from build123d import *

# Parameters (mm, degrees)
SKETCH012_W     = 64
SKETCH012_H     = 31
PAD006_DEPTH    = 3
SKETCH013_R     = 1.5
POCKET006_DEPTH = 5
SKETCH014_W     = 8
SKETCH014_H     = 6
POCKET007_DEPTH = 5


with BuildPart() as part:
    # Sketch012 → Pad006 (new body)
    with BuildSketch(Plane.XZ.offset(-30)):
        with Locations((0, -2)):
            Rectangle(SKETCH012_W, SKETCH012_H)
    extrude(amount=PAD006_DEPTH)

    # Sketch013 (on Face5 of Pad006) → Pocket006 (cut)
    with BuildSketch(Plane(origin=(0, 30, 0), x_dir=(1, 0, 0), z_dir=(0, 1, 0))):
        with Locations((28.5, 10)):
            Circle(SKETCH013_R)
        with Locations((-28.5, 10)):
            Circle(SKETCH013_R)
    extrude(amount=-POCKET006_DEPTH, mode=Mode.SUBTRACT)

    # Sketch014 (on Face5 of Pocket006) → Pocket007 (cut)
    with BuildSketch(Plane.XZ.offset(-27)):
        with Locations((19.4, -6)):
            Rectangle(SKETCH014_W, SKETCH014_H)
        with Locations((-0.5, -12)):
            Rectangle(SKETCH014_W, SKETCH014_H)
        with Locations((-19.4, -6)):
            Rectangle(SKETCH014_W, SKETCH014_H)
    extrude(amount=-POCKET007_DEPTH, mode=Mode.SUBTRACT)


with BuildPart() as part_1:
    # Body004 placement: moved
    add(part.part.moved(Location((0, -57, 0))))


solid = part_1.part
For this review, take the finished solid that the model builds, in its own axes (mm). A direction names the side the tool comes from. Round coordinates to 2 decimals unless told otherwise and drop trailing zeros. Loops run counter-clockwise (first coordinate to the right, second up) from the corner with the lowest first, then second, coordinate; pieces in that order, holes last. Notation, with made-up numbers: (-18, 55.25) - (27, 55.25) arc R21 cw to (27, 91.25) - close; hole circle Ø11 at (22.5, 53.25). An arc over 180 degrees is marked (long way). Use one line per item in the form item = value.
Item 1: Consider section D-D on y = -29.1. Write out the cut boundary in (x, z), then the cut area to 3 significant figures.
Answers:
outline = (-32, -17.5) - (32, -17.5) - (32, 13.5) - (-32, 13.5) - close; hole circle Ø3 at (-28.5, -10); hole (-23.4, -9) - (-15.4, -9) - (-15.4, -3) - (-23.4, -3) - close; hole (-4.5, -15) - (3.5, -15) - (3.5, -9) - (-4.5, -9) - close; hole (15.4, -9) - (23.4, -9) - (23.4, -3) - (15.4, -3) - close; hole circle Ø3 at (28.5, -10)
area = 1,830 mm^2
Item 2: Consider section A-A on x = -19.5. Write out the cut boundary in (y, z).
Answers:
outline = (-30, -17.5) - (-27, -17.5) - (-27, -9) - (-30, -9) - close; (-30, -3) - (-27, -3) - (-27, 13.5) - (-30, 13.5) - close
Item 3: Clearance check with a flat-ended pin moving along its axis: P1, Ø1.8, axis at x = -28.5, z = -10, coming from the +Y side. State where the tip first meets the part, or that it passes through.
Answers:
P1 = through
Item 4: For line 1 (X direction, y = -27.9, z = -10); line 2 (X direction, y = -27.6, z = -6); line 3 (Z direction, x = -17.5, y = -29.35), list the stretches that pass through material, from the lowest coordinate up.
Answers:
line_1 = -32 to -30, -27 to -4.5, 3.5 to 27, 30 to 32
line_2 = -32 to -23.4, -15.4 to 15.4, 23.4 to 32
line_3 = -17.5 to -9, -3 to 13.5
Item 5: Tool access review of faces 5 (the flat face through (0, -27, -2)), 6 (the flat face through (19, -29, -3)): name each direction out of +Z, -Z, +X, -X, +Y, -Y from which nothing blocks a thin tool from reaching the whole face with its end or side.
Answers:
face_5 = +Z, -Z, +X, -X, +Y
face_6 = +Y, -Y
Item 6: Mouldability with a two-part tool opening along Z and no side actions: class faces 1 (the flat face through (15.4, -29, -6)), 2 (the flat face through (32, -28, -2)), 3 (the flat face through (0, -28, -17.5)), 4 (the flat face through (0, -28, 13.5)) as +Z half, -Z half, draft (parallel to the pull), parting line (faces both ways), or undercut.
Answers:
face_1 = undercut
face_2 = draft
face_3 = -Z half
face_4 = +Z half
Item 7: Consider section B-B on z = -10. Write out the cut boundary in (x, y).
Answers:
outline = (-32, -30) - (-30, -30) - (-30, -27) - (-32, -27) - close; (-27, -30) - (-4.5, -30) - (-4.5, -27) - (-27, -27) - close; (3.5, -30) - (27, -30) - (27, -27) - (3.5, -27) - close; (30, -30) - (32, -30) - (32, -27) - (30, -27) - close
Item 8: Consider section C-C on z = -6.5. Write out the cut boundary in (x, y), then the cut area to 3 significant figures.
Answers:
outline = (-32, -30) - (-23.4, -30) - (-23.4, -27) - (-32, -27) - close; (-15.4, -30) - (15.4, -30) - (15.4, -27) - (-15.4, -27) - close; (23.4, -30) - (32, -30) - (32, -27) - (23.4, -27) - close
area = 144 mm^2
